from build123d import *

# Parameters (mm, degrees)
PAD_DEPTH       = 5
SKETCH001_R     = 2.1
POCKET_DEPTH    = 13.001
SKETCH002_R     = 2.1
POCKET001_DEPTH = 5
FILLET_R        = 4.9


with BuildPart() as part:
    # Sketch → Pad (new body, symmetric)
    with BuildSketch(Plane.XY):
        with BuildLine():
            Line((-6.5, -5), (-6.5, 5))
            ThreePointArc((-5, 6.5), (-6.06066, 6.06066), (-6.5, 5))
            Line((-5, 6.5), (5, 6.5))
            ThreePointArc((6.5, 5), (6.06066, 6.06066), (5, 6.5))
            Line((6.5, 5), (6.5, -5))
            Line((5.5, -5), (6.5, -5))
            Line((5.5, 4.999996), (5.5, -5))
            ThreePointArc((5.5, 4.999996), (5.353558, 5.353549), (5.000009, 5.5))
            Line((-5, 5.5), (5.000009, 5.5))
            ThreePointArc((-5, 5.5), (-5.353553, 5.353553), (-5.5, 5))
            Line((-5.5, -5), (-5.5, 5))
            Line((-6.5, -5), (-5.5, -5))
        make_face()
    extrude(amount=PAD_DEPTH, both=True)

    # Sketch001 → Pocket (cut, through all)
    with BuildSketch(Plane(origin=(-6.5, 0, 0), x_dir=(0, -1, 0), z_dir=(-1, 0, 0))):
        Circle(SKETCH001_R)
    extrude(amount=-POCKET_DEPTH, mode=Mode.SUBTRACT)

    # Sketch002 → Pocket001 (cut)
    with BuildSketch(Plane(origin=(0, 6.5, 0), x_dir=(-1, 0, 0), z_dir=(0, 1, 0))):
        Circle(SKETCH002_R)
    extrude(amount=-POCKET001_DEPTH, mode=Mode.SUBTRACT)

    # Fillet
    fillet_edges = [part.edges().sort_by_distance(p)[0] for p in [
        (-6, -5, -5),
        (6, -5, -5),
        (6, -5, 5),
        (-6, -5, 5),
    ]]
    fillet(fillet_edges, radius=FILLET_R)


solid = part.part
Can you work these out from the model? Positions are in its coordinate system, mm. A direction names the side the tool comes from. Give positions to 0.01 mm unless a question says otherwise; leave off trailing zeros. Loops run counter-clockwise (first coordinate to the right, second up) from the corner with the lowest first, then second, coordinate; pieces in that order, holes last. Notation, with made-up numbers: (-39.5, 12) - (-20.5, 12) arc R25 ccw to (-20.5, 47) - close; hole circle Ø1 at (18, 51.25). An arc over 180 degrees is marked (long way). Return JSON: item names as keys, results as strings.
1. For faces 4 (the face through (5.5, 2.3, 0.1)), 5 (the face through (0, 6, -5)), which set-ups out of +Z, -Z, +X, -X, +Y, -Y let a thin tool reach every point of the face, with its end or its side?
Output values:
{"face 4": "+Z, -Z, -Y", "face 5": "-Z, +X, -X, +Y, -Y"}
2. I'm going to push flat-ended pins straight in: pin 1 Ø6 at (x, z) = (1, -2) entering from -Y; pin 2 Ø6 at (x, z) = (-4.5, -3.5) entering from -Y. Where does each tip first touch, or does it pass through?
Output values:
{"pin 1": "stops at y = 5.5", "pin 2": "stops at y = -4.97"}
3. I want a section at D-D on y = 1.75. Please give me the cut outline in (x, z), and give its area (3 significant figures).
Output values:
{"outline": "(-6.5, -5) - (-5.5, -5) - (-5.5, -1.16) - (-6.5, -1.16) - close; (-6.5, 1.16) - (-5.5, 1.16) - (-5.5, 5) - (-6.5, 5) - close; (5.5, -5) - (6.5, -5) - (6.5, -1.16) - (5.5, -1.16) - close; (5.5, 1.16) - (6.5, 1.16) - (6.5, 5) - (5.5, 5) - close", "area": "15.4 mm²"}
4. We'd pull the mould along X, two halves only. Please class faces 1 (the face through (6.07, 6.05, 0.07)), 2 (the face through (6.01, -3.53, -3.6)), 3 (the face through (-5.5, 2.2, -1)): +X half, -X half, draft (parallel to the pull), parting line (faces both ways), or undercut.
Output values:
{"face 1": "+X half", "face 2": "draft", "face 3": "undercut"}
5. I want a section at A-A on y = 3.75. Please give me the cut outline in (x, z), and give its area (3 significant figures).
Output values:
{"outline": "(-6.5, -5) - (-5.5, -5) - (-5.5, 5) - (-6.5, 5) - close; (5.5, -5) - (6.5, -5) - (6.5, 5) - (5.5, 5) - close", "area": "20.0 mm²"}
6. I want a section at C-C on z = 1.25. Please give me the cut outline in (x, y).
Output values:
{"outline": "(-6.5, -4.86) - (-5.5, -4.86) - (-5.5, -1.69) - (-6.5, -1.69) - close; (-6.5, 1.69) - (-5.5, 1.69) - (-5.5, 5) arc R0.5 cw to (-5, 5.5) - (-1.69, 5.5) - (-1.69, 6.5) - (-5, 6.5) arc R1.5 ccw to (-6.5, 5) - close; (1.69, 5.5) - (5, 5.5) arc R0.5 cw to (5.5, 5) - (5.5, 1.69) - (6.5, 1.69) - (6.5, 5) arc R1.5 ccw to (5, 6.5) - (1.69, 6.5) - close; (5.5, -4.86) - (6.5, -4.86) - (6.5, -1.69) - (5.5, -1.69) - close"}
7. I want a section at B-B on x = 0. Please give me the cut outline in (y, z), and give its area (3 significant figures).
Output values:
{"outline": "(5.5, -5) - (6.5, -5) - (6.5, -2.1) - (5.5, -2.1) - close; (5.5, 2.1) - (6.5, 2.1) - (6.5, 5) - (5.5, 5) - close", "area": "5.80 mm²"}
8. If I drill on line 1 (Z direction, x = -5.7, y = 0); line 2 (X direction, y = 3.25, z = 2.5); line 3 (Y direction, x = -5, z = 4.5), over which ranges is the centre line in solid material (lowest first)?
Output values:
{"line 1": "z = -5 to -2.1, 2.1 to 5", "line 2": "x = -6.5 to -5.5, 5.5 to 6.5", "line 3": "y = 5.5 to 6.5"}
